Can you work these out from the model? Positions are in its coordinate system, mm. A direction names the side the tool comes from. Round coordinates to 2 decimals unless told otherwise and drop trailing zeros. Loops run counter-clockwise (first coordinate to the right, second up) from the corner with the lowest first, then second, coordinate; pieces in that order, holes last. Notation, with made-up numbers: M 23,55.25 L 76,55.25 A17 ccw 76,72.25 Z; hole C -19.5,44 d1. An arc over 180 degrees is marked long. Return JSON: item names as keys, results as strings.
```python
from build123d import *

# Parameters (mm, degrees)
F4_W     = 4.1551380418
F4_H     = 14.0508930199
F5_DEPTH = 0.5
F6_W     = 15.2522735298
F6_H     = 13.0339283496
F7_DEPTH = 12.5


with BuildPart() as f1:
    # F0 (on Front) → F1 (revolve)
    with BuildSketch(Plane.XZ):
        with BuildLine():
            Line((-0.4280307109, 11.4827230744), (-0.4261488038, 11.4827230744))
            add(Edge.make_bspline(
                [(-0.4261488038, 11.4827230744), (-0.556664915, 11.2998342577), (-0.6817765252, 11.007238571)],
                knots=[0.2242103955, 0.2242103955, 0.2242103955, 0.3636698207, 0.3636698207, 0.3636698207], degree=2, weights=[1, 0.9975698685, 1]))
            ThreePointArc((-0.6817765252, 11.007238571), (-0.7788007209, 10.9669177702), (-0.7377063806, 10.8702186661))
            add(Edge.make_bspline(
                [(-0.7377063806, 10.8702186661), (-4.1805245814, 2.0482402355), (-1.0087089855, -10.0145657089)],
                knots=[0.3950853549, 0.3950853549, 0.3950853549, 2.5873747735, 2.5873747735, 2.5873747735], degree=2, weights=[1, 0.4570286054, 1]))
            ThreePointArc((-1.0087089855, -10.0145657089), (-1.0611021421, -10.1053598506), (-0.9701333294, -10.1574491407))
            add(Edge.make_bspline(
                [(-0.9701333294, -10.1574491407), (-0.5208925622, -11.7775146313), (0, -11.7775146313)],
                knots=[2.610875288, 2.610875288, 2.610875288, 3.1415926536, 3.1415926536, 3.1415926536], degree=2, weights=[1, 0.9649984965, 1]))
            Line((0, -11.7775146313), (0, 11.4827230744))
            Line((0, 11.4827230744), (0, 11.7775146313))
            Line((0, 11.7775146313), (0, 12.6633324179))
            Line((0, 12.6633324179), (0, 14.7848022901))
            Line((0, 14.7848022901), (0, 16.4847507584))
            Line((0, 16.4847507584), (0, 16.7663060129))
            Line((0, 16.7663060129), (-0.5209763767, 16.7663060129))
            Line((-0.5209763767, 16.7663060129), (-0.5209763767, 16.4847507584))
            Line((-0.5209763767, 16.4847507584), (-0.3074016407, 16.4847507584))
            Line((-0.3074016407, 16.4847507584), (-0.3074016407, 14.7848022901))
            Line((-0.3074016407, 14.7848022901), (-0.419876547, 14.7848022901))
            Line((-0.419876547, 14.7848022901), (-0.419876547, 12.6633324179))
            Line((-0.419876547, 12.6633324179), (-0.4280307109, 12.6633324179))
            Line((-0.4280307109, 12.6633324179), (-0.4280307109, 11.4827230744))
        make_face()
    revolve(axis=Axis((0, 0, 0), (0, 0, -1)))

    # F2 (on Front) → F3 (revolve, cut)
    with BuildSketch(Plane.XZ):
        Polygon((0, 0), (0, 1.129917684), (-1.5530794626, 1.129917684), (-1.5530794626, 0), (-1.5530794626, -1.129917684), (0, -1.129917684), align=None)
    revolve(axis=Axis((0, 0, -0.564958842), (0, 0, -1)), mode=Mode.SUBTRACT)

    # F4 (on Front) → F5 (cut, symmetric)
    with BuildSketch(Plane.XZ):
        with Locations((2.0775690209, 0.1454737503)):
            Rectangle(F4_W, F4_H)
    extrude(amount=F5_DEPTH, both=True, mode=Mode.SUBTRACT)

    # F6 (on Front) → F7 (cut, symmetric)
    with BuildSketch(Plane.XZ):
        with Locations((0.2463888377, -6.5169641748)):
            Rectangle(F6_W, F6_H)
    extrude(amount=F7_DEPTH, both=True, mode=Mode.SUBTRACT)


solid = f1.part
```
Q1. On a 3-axis mill with a long thin cutter (end or side, diameter ignored), from which of +Z, -Z, +X, -X, +Y, -Y can I reach the whole of each face in a straight line? I mean faces 1 (the cylindrical face through (-1.55, -0.06, 0.56)), 2 (the flat face through (0, 0, 4)), 3 (the cylindrical face through (0.09, -0.42, 12.06)). Say none if no direction works.
Results:
{"face 1": "-Z", "face 2": "-Z, +X", "face 3": "none"}
Q2. Thinking about a two-plate mould opening in Z: for faces 4 (the cylindrical face through (0.309, 0.284, 13.709)), 5 (the flat face through (1, -0.5, 4)), 6 (the flat face through (0, 0, 16.766)), 7 (the flat face through (-0.4, 0, 1.13)), which applies, pulls with the +Z half, pulls with the -Z half, needs draft (parallel to the pull), parting line crosses it, or undercut?
Results:
{"face 4": "undercut", "face 5": "needs draft", "face 6": "pulls with the +Z half", "face 7": "pulls with the -Z half"}
Q3. Suppose I cut it at A-A, the plane z = 12. Please give me the cut outline in (x, y), plus the area to 3 significant figures.
Results:
{"outline": "C 0,0 d0.86", "area": "0.576 mm2"}
Q4. If I drill on line 1 along X through (y, z) = (0, 0.4); line 2 along Y through (x, z) = (0, 0.7); line 3 along Y through (x, z) = (0.9, 6.5), over which ranges is the centre line in solid material (lowest first)?
Results:
{"line 1": "x = -1.92 to -1.55", "line 2": "y = -1.91 to -1.55, 1.55 to 1.91", "line 3": "y = -1.32 to -0.5, 0.5 to 1.32"}
Q5. I'm going to push flat-ended pins straight in: pin 1 Ø2 at (x, z) = (1.5, 2) entering from -Y; pin 2 Ø1.9 at (x, y) = (0, 0) entering from -Z; pin 3 Ø0.9 at (x, z) = (0.5, 3) entering from +Y. Where does each tip first touch, or does it pass through?
Results:
{"pin 1": "stops at y = -1.82", "pin 2": "stops at z = 1.13", "pin 3": "stops at y = 1.86"}
